The listing builds one solid part. Answer for the finished solid, in the listing's coordinates (mm). A direction names the side the tool comes from. Give positions to 0.01 mm unless a question says otherwise; leave off trailing zeros. Loops run counter-clockwise (first coordinate to the right, second up) from the corner with the lowest first, then second, coordinate; pieces in that order, holes last. Notation, with made-up numbers: M 27.25,-9.75 L 76.25,-9.75 A31 ccw 76.25,22.25 Z; hole C 19,12 d6. An arc over 180 degrees is marked long. Return JSON: item names as keys, results as strings.
from build123d import *

# Parameters (mm, degrees)
EXTRUDE_1_DEPTH     = 35
SKETCH_2_W          = 25
SKETCH_2_H          = 20
CUT_EXTRUDE_1_DEPTH = 67.895440801


with BuildPart() as part:
    # Эскиз1 → Бобышка-Вытянуть1 (new body)
    with BuildSketch(Plane.XY):
        Polygon((35, 22.5), (-35, -22.5), (28, -22.5), (28, -6.5), (35, 13.5), align=None)
    extrude_1 = extrude(amount=EXTRUDE_1_DEPTH)

    # Эскиз2 → Вырез-Вытянуть1 (cut, through all)
    with BuildSketch(Plane.XZ.offset(22.5)):
        with Locations((-22.5, 17.5)):
            Rectangle(SKETCH_2_W, SKETCH_2_H)
    cut_extrude_1 = extrude(amount=-CUT_EXTRUDE_1_DEPTH, mode=Mode.SUBTRACT)

    # Зеркальное отражение1: Бобышка-Вытянуть1, Вырез-Вытянуть1 across plane
    add(extrude_1.mirror(Plane(origin=(35, 0, 35), x_dir=(0, 0, 1), z_dir=(-1, 0, 0))))
    add(cut_extrude_1.mirror(Plane(origin=(35, 0, 35), x_dir=(0, 0, 1), z_dir=(-1, 0, 0))), mode=Mode.SUBTRACT)


solid = part.part
(1) A tool of negligible diameter and unlimited length cuts with its end or side. For faces 4 (the flat face through (80, -15, 17)), 5 (the flat face through (-17, -18, 7.5)), 6 (the flat face through (28, -15, 17)), from which of +Z, -Z, +X, -X, +Y, -Y can it reach the whole face along a straight path? Write none if from no direction.
Values follow:
{"face 4": "+X, +Y, -Y", "face 5": "-X, +Y, -Y", "face 6": "+Z, -Z, -Y"}
(2) Straight lines are drawn through the part: line 1 along X through (y, z) = (-7, 19.5); line 2 along X through (y, z) = (11, 4.5) (3 decimals); line 3 along Y through (x, z) = (20.5, 28). For each, find the intervals that lie inside material, in ascending order.
Values follow:
{"line 1": "-10 to 28, 42 to 80", "line 2": "17.111 to 34.125, 35.875 to 52.889", "line 3": "-22.5 to 13.18"}
(3) The part is cut by section C-C (x = 92). Determine the outline of the cut face in (y, z).
Values follow:
{"outline": "M -22.5,0 L -14.14,0 L -14.14,7.5 L -22.5,7.5 Z; M -22.5,27.5 L -14.14,27.5 L -14.14,35 L -22.5,35 Z"}
(4) The part is cut by section D-D (z = 3). Determine the outline of the cut face in (x, y), and give its area (3 significant figures).
Values follow:
{"outline": "M -35,-22.5 L 28,-22.5 L 28,-6.5 L 35,13.5 L 42,-6.5 L 42,-22.5 L 105,-22.5 L 35,22.5 Z", "area": "2,790 mm²"}
(5) Determine the mould class of faces 1 (the flat face through (42, -15, 17)), 2 (the flat face through (20, -10, 0)), 3 (the flat face through (61.732, 5.315, 17.255)) for opening direction X: released by +X, released by -X, zero draft, split by the parting line, or undercut.
Values follow:
{"face 1": "undercut", "face 2": "zero draft", "face 3": "released by +X"}
(6) Given pin 1 (10 mm diameter, centred on y = -6.5, z = 3.5, fed in from -X); pin 2 (6 mm diameter, centred on x = 25, z = 8.5, fed in from +Y); pin 3 (17.5 mm diameter, centred on y = -12.5, z = 21.5, fed in from +X), each flat-ended and moving along its own axis, determine where each tip first touches the part or whether it passes through.
Values follow:
{"pin 1": "x = -17.89", "pin 2": "y = 18", "pin 3": "x = 99.35"}
(7) The part is cut by section B-B (y = 11). Determine the outline of the cut face in (x, z) (3 decimals).
Values follow:
{"outline": "M 17.111,0 L 34.125,0 L 34.125,35 L 17.111,35 Z; M 35.875,0 L 52.889,0 L 52.889,35 L 35.875,35 Z"}
(8) The part is cut by section A-A (z = 9). Determine the outline of the cut face in (x, y).
Values follow:
{"outline": "M -10,-22.5 L 28,-22.5 L 28,-6.5 L 35,13.5 L 42,-6.5 L 42,-22.5 L 80,-22.5 L 80,-6.43 L 35,22.5 L -10,-6.43 Z"}
